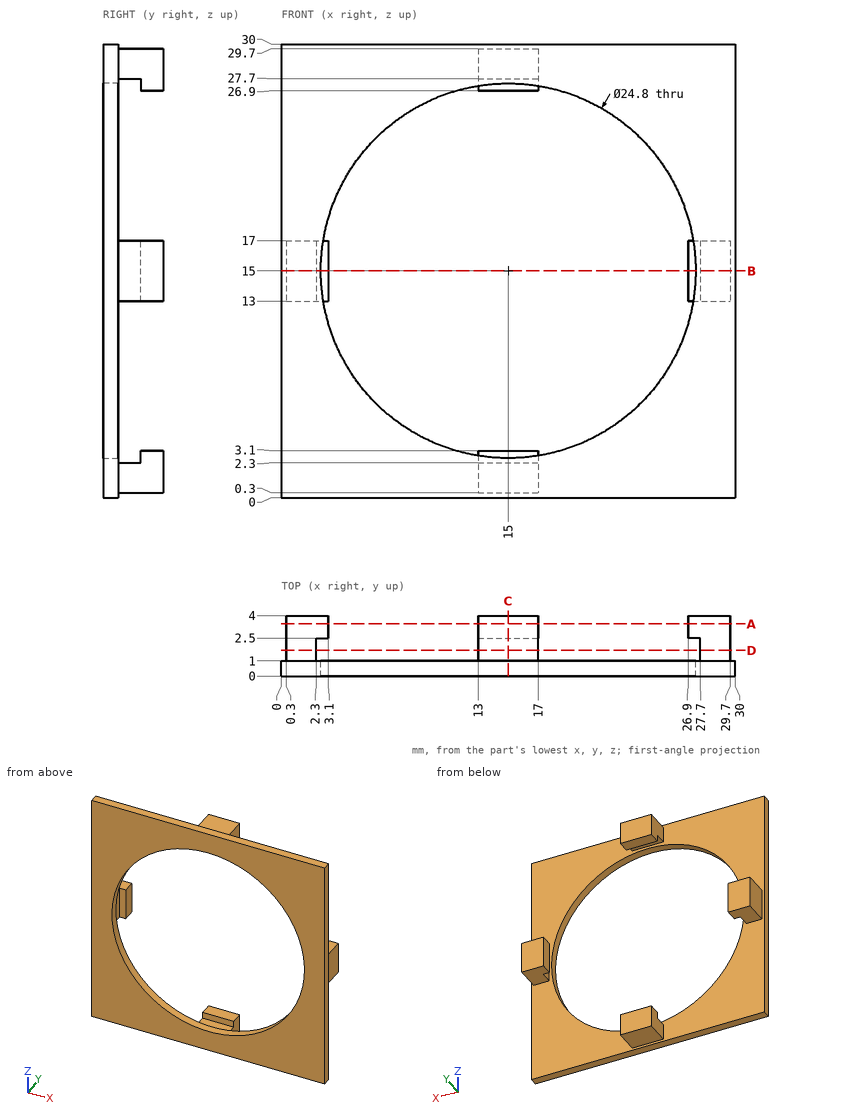
Could you check a few things on this drawing? It's one solid part, dimensions in mm from its lowest x, y, z. Round coordinates to 2 decimals unless told otherwise and drop trailing zeros. Order: outer loops, then holes, each group sorted by start corner. A loop starts at its lowest first (then second) coordinate and runs counter-clockwise, first axis right, second up. Notation, with made-up numbers: M -12.5,79 L 14.5,79 A25 cw 14.5,92 Z; hole C 64,76.5 d9. An arc over 180 degrees is marked long. Return JSON: item names as keys, results as strings. Group by question number.
1. If we section it at A-A on y = 3.45: List the corners of the cut face in (x, z) for me.
2. I'm going to push flat-ended pins straight in: pin 1 Ø1.4 at (x, y) = (1, 2) entering from -Z; pin 2 Ø0.8 at (x, y) = (1.5, 2) entering from +Z; pin 3 Ø0.8 at (y, z) = (3.5, 14.5) entering from -X. Where does each tip first touch, or does it pass through?
3. If we section it at C-C on x = 15: List the corners of the cut face in (y, z) for me, then the cut area to 3 significant figures.
4. Please list where these lines run through material, in increasing order: probe 1 along X at (y, z) = (0.65, 15); probe 2 along Y at (x, z) = (16, 2.5); probe 3 along X at (y, z) = (1.55, 14.5).
5. If we section it at B-B on z = 15: List the corners of the cut face in (x, y) for me, then the cut area to 3 significant figures.
6. If we section it at D-D on y = 1.7: List the corners of the cut face in (x, z) for me, then the cut area to 3 significant figures.
Reply:
{
 "1": {"outline": "M 0.3,13 L 3.1,13 L 3.1,17 L 0.3,17 Z; M 13,0.3 L 17,0.3 L 17,3.1 L 13,3.1 Z; M 13,26.9 L 17,26.9 L 17,29.7 L 13,29.7 Z; M 26.9,13 L 29.7,13 L 29.7,17 L 26.9,17 Z"},
 "2": {"pin 1": "z = 13", "pin 2": "z = 17", "pin 3": "x = 0.3"},
 "3": {"outline": "M 0,0 L 1,0 L 1,0.3 L 4,0.3 L 4,3.1 L 2.5,3.1 L 2.5,2.3 L 1,2.3 L 1,2.6 L 0,2.6 Z; M 0,27.4 L 1,27.4 L 1,27.7 L 2.5,27.7 L 2.5,26.9 L 4,26.9 L 4,29.7 L 1,29.7 L 1,30 L 0,30 Z", "area": "19.6 mm^2"},
 "4": {"probe 1": "0 to 2.6, 27.4 to 30", "probe 2": "0 to 1, 2.5 to 4", "probe 3": "0.3 to 2.3, 27.7 to 29.7"},
 "5": {"outline": "M 0,0 L 2.6,0 L 2.6,1 L 2.3,1 L 2.3,2.5 L 3.1,2.5 L 3.1,4 L 0.3,4 L 0.3,1 L 0,1 Z; M 26.9,2.5 L 27.7,2.5 L 27.7,1 L 27.4,1 L 27.4,0 L 30,0 L 30,1 L 29.7,1 L 29.7,4 L 26.9,4 Z", "area": "19.6 mm^2"},
 "6": {"outline": "M 0.3,13 L 2.3,13 L 2.3,17 L 0.3,17 Z; M 13,0.3 L 17,0.3 L 17,2.3 L 13,2.3 Z; M 13,27.7 L 17,27.7 L 17,29.7 L 13,29.7 Z; M 27.7,13 L 29.7,13 L 29.7,17 L 27.7,17 Z", "area": "32.0 mm^2"}
}
